```python
from build123d import *

# Parameters (mm, degrees)
SKETCH1_W            = 130
SKETCH1_H            = 63
BOSS_EXTRUDE1_DEPTH  = 15
LPATTERN1_COUNT      = 2
LPATTERN1_PITCH      = 46.5
LPATTERN1_COUNT_DIR2 = 2
LPATTERN1_PITCH_DIR2 = 46.5
LPATTERN2_COUNT      = 2
LPATTERN2_PITCH      = 100
LPATTERN2_COUNT_DIR2 = 2
LPATTERN2_PITCH_DIR2 = 46.5
SKETCH6_R            = 10
BOSS_EXTRUDE2_DEPTH  = 588
SKETCH7_R            = 10
BOSS_EXTRUDE3_DEPTH  = 588
SKETCH10_W           = 40
SKETCH10_H           = 40
SKETCH10_W_2         = 18
SKETCH10_H_2         = 30
CUT_EXTRUDE1_DEPTH   = 10
SKETCH11_R           = 2.5
CUT_EXTRUDE2_DEPTH   = 16


with BuildPart() as part:
    # Sketch1 → Boss-Extrude1 (new body)
    with BuildSketch(Plane.XY.offset(89)):
        Rectangle(SKETCH1_W, SKETCH1_H)
    extrude(amount=-BOSS_EXTRUDE1_DEPTH)

    # Sketch2 → Cut-Revolve1 (revolve, cut)
    with BuildSketch(Plane(origin=(23.25, 0, 0), x_dir=(0, 0, -1), z_dir=(1, 0, 0))):
        Polygon((-89, 23.25), (-89, 27.25), (-88.3235, 26.5735), (-74.6765, 26.5735), (-74, 27.25), (-74, 23.25), align=None)
    cut_revolve1 = revolve(axis=Axis((23.25, 23.25, 74), (0, 0, 1)), mode=Mode.SUBTRACT)

    # LPattern1: Cut-Revolve1 2 × 2
    with Locations(*[(-i * LPATTERN1_PITCH, -j * LPATTERN1_PITCH_DIR2, 0) for i in range(LPATTERN1_COUNT) for j in range(LPATTERN1_COUNT_DIR2) if (i, j) != (0, 0)]):
        add(cut_revolve1, mode=Mode.SUBTRACT)

    # Sketch4 → Cut-Revolve2 (revolve, cut)
    with BuildSketch(Plane(origin=(50, 0, 0), x_dir=(0, 0, -1), z_dir=(1, 0, 0))):
        Polygon((-89, 23.25), (-89, 27.75), (-83, 27.75), (-83, 30.75), (-74, 30.75), (-74, 23.25), align=None)
    cut_revolve2 = revolve(axis=Axis((50, 23.25, 74), (0, 0, 1)), mode=Mode.SUBTRACT)

    # LPattern2: Cut-Revolve2 2 × 2
    with Locations(*[(-i * LPATTERN2_PITCH, -j * LPATTERN2_PITCH_DIR2, 0) for i in range(LPATTERN2_COUNT) for j in range(LPATTERN2_COUNT_DIR2) if (i, j) != (0, 0)]):
        add(cut_revolve2, mode=Mode.SUBTRACT)

    # Sketch6 → Boss-Extrude2 (add)
    with BuildSketch(Plane.XY.offset(89)):
        with Locations((-52, 0)):
            Circle(SKETCH6_R)
    extrude(amount=-BOSS_EXTRUDE2_DEPTH)

    # Sketch7 → Boss-Extrude3 (add)
    with BuildSketch(Plane.XY.offset(89)):
        with Locations((52, 0)):
            Circle(SKETCH7_R)
    extrude(amount=-BOSS_EXTRUDE3_DEPTH)

    # Sketch8 → Revolve1 (revolve)
    with BuildSketch(Plane(origin=(0, 0, 0), x_dir=(0, 0, -1), z_dir=(1, 0, 0))):
        Polygon((-74, 0), (-74, 30), (-60.6, 30), (-59, 28.4), (-59, 11), (-50, 11), (-49, 10), (-49, 0), align=None)
    revolve(axis=Axis((0, 0, 49), (0, 0, 1)))

    # Sketch9 → Cut-Revolve3 (revolve, cut)
    with BuildSketch(Plane(origin=(0, 0, 0), x_dir=(0, 0, -1), z_dir=(1, 0, 0))):
        Polygon((-74, 0), (-74, 7.188), (-49.812, 7.188), (-49, 8), (-49, 0), align=None)
    revolve(axis=Axis((0, 0, 49), (0, 0, 1)), mode=Mode.SUBTRACT)

    # Sketch10 → Cut-Extrude1 (cut)
    with BuildSketch(Plane.XY.offset(49)):
        Rectangle(SKETCH10_W, SKETCH10_H)
        Rectangle(SKETCH10_W_2, SKETCH10_H_2, mode=Mode.SUBTRACT)
    extrude(amount=CUT_EXTRUDE1_DEPTH, mode=Mode.SUBTRACT)

    # Sketch11 → Cut-Extrude2 (cut, through all)
    with BuildSketch(Plane(origin=(0, 0, 74), x_dir=(-1, 0, 0), z_dir=(0, 0, -1))):
        with Locations((-59, 14.25)):
            Circle(SKETCH11_R)
        with Locations((59, -14.25)):
            Circle(SKETCH11_R)
    extrude(amount=-CUT_EXTRUDE2_DEPTH, mode=Mode.SUBTRACT)


solid = part.part
```
Design review of the part built by this model. Coordinates are the model's own, in mm. A direction names the side the tool comes from. Round coordinates to 2 decimals unless told otherwise and drop trailing zeros. Write each loop counter-clockwise with the first axis right and the second up, starting at its lowest first coordinate (ties: lowest second). Pieces come first, ordered by that corner, then holes. Notation, with made-up numbers: (0, 78) -> (24, 78) arc R15 ccw to (24, 87) -> close; hole circle Ø8 at (20, 27). An arc over 180 degrees is marked (long way). Write item = value, one per line. Start each with the question number.
1) Mouldability with a two-part tool opening along X and no side actions: class faces 1 (the face through (9, 0, 54)), 2 (the face through (-1, 0, 89)), 3 (the face through (-65, 0, 82)) as +X half, -X half, draft (parallel to the pull), parting line (faces both ways), or undercut.
2) Take a section at B-B, the plane x = 0. State the section outline as (y, z) points.
3) Clearance check with flat-ended pins moving along their axes: pin 1 (9 mm diameter, centred on x = -1.5, y = 4, fed in from -Z); pin 2 (10.5 mm diameter, centred on x = -50, y = 23.25, fed in from -Z); pin 3 (3 mm diameter, centred on x = -20, y = 21.5, fed in from +Z); pin 4 (3 mm diameter, centred on x = -44, y = 15.5, fed in from -Z). State where each tip first meets the part, or that it passes through.
4) Tool access review of faces 4 (the face through (-7.127, -0.936, 61.737)), 5 (the face through (-9, 0, 54)), 6 (the face through (-1, -31.5, 82)): name each direction out of +Z, -Z, +X, -X, +Y, -Y from which nothing blocks a thin tool from reaching the whole face with its end or side.
5) Wall thickness on probe 1 along X at (y, z) = (23, 85); probe 2 along Y at (x, z) = (-50, 86.9); probe 3 along X at (y, z) = (-23, 79): over which ranges is each line inside the solid? List them lowest first. Write a range as from..to.
6) Take a section at A-A, the plane z = -267. State the section outline as (x, y) points, plus the area to 3 significant figures.
Results list:
q1.face_1 = undercut
q1.face_2 = draft
q1.face_3 = -X half
q2.outline = (-31.5, 74) -> (-30, 74) -> (-30, 60.6) -> (-28.4, 59) -> (-11, 59) -> (-11, 50) -> (-10, 49) -> (-8, 49) -> (-7.19, 49.81) -> (-7.19, 74) -> (7.19, 74) -> (7.19, 49.81) -> (8, 49) -> (10, 49) -> (11, 50) -> (11, 59) -> (28.4, 59) -> (30, 60.6) -> (30, 74) -> (31.5, 74) -> (31.5, 89) -> (-31.5, 89) -> close
q3.pin_1 = 49
q3.pin_2 = 83
q3.pin_3 = 89
q3.pin_4 = 74
q4.face_4 = -Z
q4.face_5 = -Z, +Y, -Y
q4.face_6 = +Z, -Z, +X, -X, -Y
q5.probe_1 = -65..-54.49, -45.51..-26.56, -19.94..19.94, 26.56..45.51, 54.49..65
q5.probe_2 = -31.5..-27.75, -18.75..18.75, 27.75..31.5
q5.probe_3 = -65..-57.5, -42.5..-26.56, -19.94..19.94, 26.56..42.5, 57.5..65
q6.outline = circle Ø20 at (-52, 0); circle Ø20 at (52, 0)
q6.area = 628 mm²
